The listing builds one solid part. Answer for the finished solid, in the listing's coordinates (mm). Face numbers are marked on the shaded views. A direction names the side the tool comes from. Give positions to 0.01 mm unless a question says otherwise; leave off trailing zeros. Order: outer loops, then holes, each group sorted by start corner. A loop starts at its lowest first (then second) coordinate and runs counter-clockwise, first axis right, second up. Notation, with made-up numbers: (0, 55.25) - (19, 55.25) arc R7 cw to (19, 65.25) - close; hole circle Ø2 at (11, 59). An arc over 180 degrees is marked (long way). Write each question's results on one line, items separated by ' | '. Start each with the question number.
1. Section A-A (z = 1.1) is taken. Give the vertices of the cut face in (x, y), and give its area (3 significant figures).
2. Find the intervals of material crossed by L1, parallel to X at y = -351.5, z = 2.45; L2, parallel to Y at x = 74.5, z = 1.1; L3, parallel to X at y = -365, z = 0.2, in increasing order.
3. Which of the six approach directions +Z, -Z, +X, -X, +Y, -Y give full straight-line access (tool end or side, diameter ignored) to the marked faces 4 and 5?
4. Determine the mould class of the marked faces 1, 2 and 3 for opening direction X: released by +X, released by -X, zero draft, split by the parting line, or undercut.
5. Flat-ended cylindrical pins translate along their axes: pin 1 (2 mm diameter, centred on x = 73.59, y = -350.57, fed in from +Z); pin 2 (1.5 mm diameter, centred on x = 65, z = 1, fed in from +Y); pin 3 (1.5 mm diameter, centred on y = -356.5, z = 1, fed in from -X). Find the tip coordinate at first contact, or state that the pin passes through.
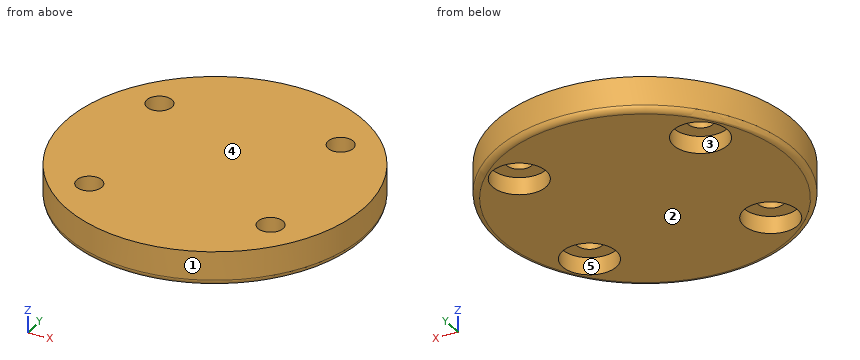
from build123d import *

# Parameters (mm, degrees)
SKETCH_1_R          = 13
SKETCH_1_R_2        = 1.1
EXTRUDE_1_DEPTH     = 3
FILLET_1_R          = 0.5
SKETCH_2_R          = 2.35
CUT_EXTRUDE_1_DEPTH = 1.5


with BuildPart() as part:
    # 草图1 → 凸台-拉伸1 (new body)
    with BuildSketch(Plane.XY):
        with Locations((66.770274295, -357.783074412)):
            Circle(SKETCH_1_R)
        with Locations((59.955130925, -364.997907801)):
            Circle(SKETCH_1_R_2, mode=Mode.SUBTRACT)
        with Locations((74.880510465, -363.503569956)):
            Circle(SKETCH_1_R_2, mode=Mode.SUBTRACT)
        with Locations((58.660038126, -352.062578867)):
            Circle(SKETCH_1_R_2, mode=Mode.SUBTRACT)
        with Locations((73.585417665, -350.568241022)):
            Circle(SKETCH_1_R_2, mode=Mode.SUBTRACT)
    extrude(amount=EXTRUDE_1_DEPTH)

    # 圆角1
    fillet_1_edges = [part.edges().sort_by_distance(p)[0] for p in [
        (53.770274295, -357.783074412, 0),
    ]]
    fillet(fillet_1_edges, radius=FILLET_1_R)

    # 草图2 → 切除-拉伸1 (cut)
    with BuildSketch(Plane(origin=(0, 0, 0), x_dir=(-1, 0, 0), z_dir=(0, 0, -1))):
        with Locations((-73.585417665, -350.568241022)):
            Circle(SKETCH_2_R)
        with Locations((-58.660038126, -352.062578867)):
            Circle(SKETCH_2_R)
        with Locations((-59.955130925, -364.997907801)):
            Circle(SKETCH_2_R)
        with Locations((-74.880510465, -363.503569956)):
            Circle(SKETCH_2_R)
    extrude(amount=-CUT_EXTRUDE_1_DEPTH, mode=Mode.SUBTRACT)


solid = part.part
Reported:
1) outline: circle Ø26 at (66.77, -357.78); hole circle Ø4.7 at (58.66, -352.06); hole circle Ø4.7 at (59.96, -365); hole circle Ø4.7 at (73.59, -350.57); hole circle Ø4.7 at (74.88, -363.5) | area: 462 mm²
2) L1: 55.39 to 57.71, 59.61 to 73, 74.17 to 78.15 | L2: -368.24 to -365.82, -361.18 to -352.73, -348.4 to -347.33 | L3: 56.08 to 57.61, 62.31 to 73.07, 76.69 to 77.46
3) face 4: +Z, +X, -X, +Y, -Y | face 5: -Z
4) face 1: split by the parting line | face 2: zero draft | face 3: undercut
5) pin 1: through | pin 2: y = -344.82 | pin 3: x = 53.78
